The listing builds one solid part. Answer for the finished solid, in the listing's coordinates (mm). A direction names the side the tool comes from. Give positions to 0.01 mm unless a question says otherwise; leave off trailing zeros. Loops run counter-clockwise (first coordinate to the right, second up) from the corner with the lowest first, then second, coordinate; pieces in that order, holes last.
Item 1: A tool of negligible diameter and unlimited length cuts with its end or side. For faces 4 (the face through (2, 34, -2)), 5 (the face through (185.6, 108, -2)), 6 (the face through (205.6, 87, -2)), from which of +Z, -Z, +X, -X, +Y, -Y can it reach the whole face along a straight path? Write none if from no direction.
Item 2: Section B-B, the plane y = 60.12 is taken. Give the vertices of the cut face in (x, z), and give its area (3 significant figures).
Item 3: Section D-D, the plane y = 85 is taken. Give the vertices of the cut face in (x, z).
Item 4: Section C-C, the plane x = 152.65 is taken. Give the vertices of the cut face in (y, z).
Item 5: Section A-A, the plane x = 114 is taken. Give the vertices of the cut face in (y, z), and give its area (3 significant figures).
Item 6: Consider line 1 along X through (y, z) = (55, -2.8); line 2 along X through (y, z) = (101, -1.85); line 3 along X through (y, z) = (92, -0.65). Determine where each line is inside the solid, lowest interval first.
Item 7: The mould has two halves that part along X. Classify faces 1 (the face through (161.6, 108, -2)), 2 (the face through (197, 110, -2)), 3 (the face through (205.6, 23, -2)): pulls with the +X half, pulls with the -X half, needs draft (parallel to the pull), parting line crosses it, or undercut.
Item 8: Each of these flat-tipped pins is pushed along its axis until it touches: pin 1 Ø1.8 at (x, z) = (31, -1.5) entering from -Y; pin 2 Ø1.8 at (x, z) = (1, -1.5) entering from -Y; pin 3 Ø12 at (x, y) = (29.5, 20) entering from +Z; pin 4 Ø1.8 at (x, z) = (171.5, -2) entering from +Y. Where does it stop, or does it pass through?
from build123d import *

# Parameters (mm, degrees)
SKETCH_1_W             = 209.2
SKETCH_1_H             = 110
SM_BASE_FLANGE_1_DEPTH = 3.6
CUT_EXTRUDE_1_REACH    = 238.384
SKETCH_6_W             = 42
SKETCH_6_H             = 21
CUT_EXTRUDE_2_REACH    = 238.384
SKETCH_7_W             = 3.6
SKETCH_7_H             = 22
SKETCH_7_W_2           = 24
SKETCH_7_H_2           = 3.6
SKETCH_7_W_3           = 26
SKETCH_8_R             = 1.6
CUT_EXTRUDE_3_DEPTH    = 10
CUT_EXTRUDE_4_REACH    = 238.384
SKETCH_9_R             = 2.1


# Sheet-metal steps are written as plain solids
with BuildPart() as part:
    # Sketch 1 → Базовая кромка1 (new body)
    with BuildSketch(Plane.XY):
        with Locations((104.6, 55)):
            Rectangle(SKETCH_1_W, SKETCH_1_H)
        with BuildLine():
            Line((17, 12), (139.2, 12))
            ThreePointArc((139.2, 12), (142.735533906, 13.464466094), (144.2, 17))
            Line((144.2, 17), (144.2, 93))
            ThreePointArc((144.2, 93), (142.735533906, 96.535533906), (139.2, 98))
            Line((139.2, 98), (17, 98))
            ThreePointArc((17, 98), (13.464466094, 96.535533906), (12, 93))
            Line((12, 93), (12, 17))
            ThreePointArc((12, 17), (13.464466094, 13.464466094), (17, 12))
        make_face(mode=Mode.SUBTRACT)
    extrude(amount=-SM_BASE_FLANGE_1_DEPTH)

    # Эскиз6 → Вырез-Вытянуть1 (cut, up to next)
    with BuildSketch(Plane.XY, mode=Mode.PRIVATE) as cut_extrude_1_sk1:
        with Locations((176.7, 55)):
            Rectangle(SKETCH_6_W, SKETCH_6_H)
    cut_extrude_1_tool1 = extrude(cut_extrude_1_sk1.sketch, amount=-CUT_EXTRUDE_1_REACH, mode=Mode.PRIVATE) & part.part
    add(cut_extrude_1_tool1.solids().sort_by_distance((176.7, 55, 0))[0], mode=Mode.SUBTRACT)

    # Эскиз7 → Вырез-Вытянуть2 (cut, up to next)
    with BuildSketch(Plane(origin=(0, 0, -3.6), x_dir=(-1, 0, 0), z_dir=(0, 0, -1)), mode=Mode.PRIVATE) as cut_extrude_2_sk1:
        with Locations((-1.8, 87)):
            Rectangle(SKETCH_7_W, SKETCH_7_H)
    cut_extrude_2_tool1 = extrude(cut_extrude_2_sk1.sketch, amount=-CUT_EXTRUDE_2_REACH, mode=Mode.PRIVATE) & part.part
    # Эскиз7 → Вырез-Вытянуть2 (cut, up to next)
    with BuildSketch(Plane(origin=(0, 0, -3.6), x_dir=(-1, 0, 0), z_dir=(0, 0, -1)), mode=Mode.PRIVATE) as cut_extrude_2_sk2:
        with Locations((-35.6, 108.2)):
            Rectangle(SKETCH_7_W_2, SKETCH_7_H_2)
    cut_extrude_2_tool2 = extrude(cut_extrude_2_sk2.sketch, amount=-CUT_EXTRUDE_2_REACH, mode=Mode.PRIVATE) & part.part
    # Эскиз7 → Вырез-Вытянуть2 (cut, up to next)
    with BuildSketch(Plane(origin=(0, 0, -3.6), x_dir=(-1, 0, 0), z_dir=(0, 0, -1)), mode=Mode.PRIVATE) as cut_extrude_2_sk3:
        with Locations((-104.6, 108.2)):
            Rectangle(SKETCH_7_W_3, SKETCH_7_H_2)
    cut_extrude_2_tool3 = extrude(cut_extrude_2_sk3.sketch, amount=-CUT_EXTRUDE_2_REACH, mode=Mode.PRIVATE) & part.part
    # Эскиз7 → Вырез-Вытянуть2 (cut, up to next)
    with BuildSketch(Plane(origin=(0, 0, -3.6), x_dir=(-1, 0, 0), z_dir=(0, 0, -1)), mode=Mode.PRIVATE) as cut_extrude_2_sk4:
        with Locations((-173.6, 108.2)):
            Rectangle(SKETCH_7_W_2, SKETCH_7_H_2)
    cut_extrude_2_tool4 = extrude(cut_extrude_2_sk4.sketch, amount=-CUT_EXTRUDE_2_REACH, mode=Mode.PRIVATE) & part.part
    # Эскиз7 → Вырез-Вытянуть2 (cut, up to next)
    with BuildSketch(Plane(origin=(0, 0, -3.6), x_dir=(-1, 0, 0), z_dir=(0, 0, -1)), mode=Mode.PRIVATE) as cut_extrude_2_sk5:
        with Locations((-207.4, 87)):
            Rectangle(SKETCH_7_W, SKETCH_7_H)
    cut_extrude_2_tool5 = extrude(cut_extrude_2_sk5.sketch, amount=-CUT_EXTRUDE_2_REACH, mode=Mode.PRIVATE) & part.part
    # Эскиз7 → Вырез-Вытянуть2 (cut, up to next)
    with BuildSketch(Plane(origin=(0, 0, -3.6), x_dir=(-1, 0, 0), z_dir=(0, 0, -1)), mode=Mode.PRIVATE) as cut_extrude_2_sk6:
        with Locations((-207.4, 23)):
            Rectangle(SKETCH_7_W, SKETCH_7_H)
    cut_extrude_2_tool6 = extrude(cut_extrude_2_sk6.sketch, amount=-CUT_EXTRUDE_2_REACH, mode=Mode.PRIVATE) & part.part
    # Эскиз7 → Вырез-Вытянуть2 (cut, up to next)
    with BuildSketch(Plane(origin=(0, 0, -3.6), x_dir=(-1, 0, 0), z_dir=(0, 0, -1)), mode=Mode.PRIVATE) as cut_extrude_2_sk7:
        with Locations((-173.6, 1.8)):
            Rectangle(SKETCH_7_W_2, SKETCH_7_H_2)
    cut_extrude_2_tool7 = extrude(cut_extrude_2_sk7.sketch, amount=-CUT_EXTRUDE_2_REACH, mode=Mode.PRIVATE) & part.part
    # Эскиз7 → Вырез-Вытянуть2 (cut, up to next)
    with BuildSketch(Plane(origin=(0, 0, -3.6), x_dir=(-1, 0, 0), z_dir=(0, 0, -1)), mode=Mode.PRIVATE) as cut_extrude_2_sk8:
        with Locations((-104.6, 1.8)):
            Rectangle(SKETCH_7_W_3, SKETCH_7_H_2)
    cut_extrude_2_tool8 = extrude(cut_extrude_2_sk8.sketch, amount=-CUT_EXTRUDE_2_REACH, mode=Mode.PRIVATE) & part.part
    # Эскиз7 → Вырез-Вытянуть2 (cut, up to next)
    with BuildSketch(Plane(origin=(0, 0, -3.6), x_dir=(-1, 0, 0), z_dir=(0, 0, -1)), mode=Mode.PRIVATE) as cut_extrude_2_sk9:
        with Locations((-35.6, 1.8)):
            Rectangle(SKETCH_7_W_2, SKETCH_7_H_2)
    cut_extrude_2_tool9 = extrude(cut_extrude_2_sk9.sketch, amount=-CUT_EXTRUDE_2_REACH, mode=Mode.PRIVATE) & part.part
    # Эскиз7 → Вырез-Вытянуть2 (cut, up to next)
    with BuildSketch(Plane(origin=(0, 0, -3.6), x_dir=(-1, 0, 0), z_dir=(0, 0, -1)), mode=Mode.PRIVATE) as cut_extrude_2_sk10:
        with Locations((-1.8, 23)):
            Rectangle(SKETCH_7_W, SKETCH_7_H)
    cut_extrude_2_tool10 = extrude(cut_extrude_2_sk10.sketch, amount=-CUT_EXTRUDE_2_REACH, mode=Mode.PRIVATE) & part.part
    add(cut_extrude_2_tool1.solids().sort_by_distance((1.8, 87, -3.6))[0], mode=Mode.SUBTRACT)
    add(cut_extrude_2_tool2.solids().sort_by_distance((35.6, 108.2, -3.6))[0], mode=Mode.SUBTRACT)
    add(cut_extrude_2_tool3.solids().sort_by_distance((104.6, 108.2, -3.6))[0], mode=Mode.SUBTRACT)
    add(cut_extrude_2_tool4.solids().sort_by_distance((173.6, 108.2, -3.6))[0], mode=Mode.SUBTRACT)
    add(cut_extrude_2_tool5.solids().sort_by_distance((207.4, 87, -3.6))[0], mode=Mode.SUBTRACT)
    add(cut_extrude_2_tool6.solids().sort_by_distance((207.4, 23, -3.6))[0], mode=Mode.SUBTRACT)
    add(cut_extrude_2_tool7.solids().sort_by_distance((173.6, 1.8, -3.6))[0], mode=Mode.SUBTRACT)
    add(cut_extrude_2_tool8.solids().sort_by_distance((104.6, 1.8, -3.6))[0], mode=Mode.SUBTRACT)
    add(cut_extrude_2_tool9.solids().sort_by_distance((35.6, 1.8, -3.6))[0], mode=Mode.SUBTRACT)
    add(cut_extrude_2_tool10.solids().sort_by_distance((1.8, 23, -3.6))[0], mode=Mode.SUBTRACT)

    # Эскиз8 → Вырез-Вытянуть3 (cut)
    with BuildSketch(Plane(origin=(0, 0, -3.6), x_dir=(-1, 0, 0), z_dir=(0, 0, -1))):
        with Locations((-200.2, 9)):
            Circle(SKETCH_8_R)
        with Locations((-9, 9)):
            Circle(SKETCH_8_R)
        with Locations((-9, 101)):
            Circle(SKETCH_8_R)
        with Locations((-200.2, 101)):
            Circle(SKETCH_8_R)
    extrude(amount=-CUT_EXTRUDE_3_DEPTH, mode=Mode.SUBTRACT)

    # Эскиз9 → Вырез-Вытянуть4 (cut, up to next)
    with BuildSketch(Plane(origin=(0, 0, -3.6), x_dir=(-1, 0, 0), z_dir=(0, 0, -1)), mode=Mode.PRIVATE) as cut_extrude_4_sk1:
        with Locations((-200.91, 60.12)):
            Circle(SKETCH_9_R)
    cut_extrude_4_tool1 = extrude(cut_extrude_4_sk1.sketch, amount=-CUT_EXTRUDE_4_REACH, mode=Mode.PRIVATE) & part.part
    # Эскиз9 → Вырез-Вытянуть4 (cut, up to next)
    with BuildSketch(Plane(origin=(0, 0, -3.6), x_dir=(-1, 0, 0), z_dir=(0, 0, -1)), mode=Mode.PRIVATE) as cut_extrude_4_sk2:
        with Locations((-200.91, 49.96)):
            Circle(SKETCH_9_R)
    cut_extrude_4_tool2 = extrude(cut_extrude_4_sk2.sketch, amount=-CUT_EXTRUDE_4_REACH, mode=Mode.PRIVATE) & part.part
    # Эскиз9 → Вырез-Вытянуть4 (cut, up to next)
    with BuildSketch(Plane(origin=(0, 0, -3.6), x_dir=(-1, 0, 0), z_dir=(0, 0, -1)), mode=Mode.PRIVATE) as cut_extrude_4_sk3:
        with Locations((-152.65, 60.12)):
            Circle(SKETCH_9_R)
    cut_extrude_4_tool3 = extrude(cut_extrude_4_sk3.sketch, amount=-CUT_EXTRUDE_4_REACH, mode=Mode.PRIVATE) & part.part
    # Эскиз9 → Вырез-Вытянуть4 (cut, up to next)
    with BuildSketch(Plane(origin=(0, 0, -3.6), x_dir=(-1, 0, 0), z_dir=(0, 0, -1)), mode=Mode.PRIVATE) as cut_extrude_4_sk4:
        with Locations((-152.65, 49.96)):
            Circle(SKETCH_9_R)
    cut_extrude_4_tool4 = extrude(cut_extrude_4_sk4.sketch, amount=-CUT_EXTRUDE_4_REACH, mode=Mode.PRIVATE) & part.part
    add(cut_extrude_4_tool1.solids().sort_by_distance((200.91, 60.12, -3.6))[0], mode=Mode.SUBTRACT)
    add(cut_extrude_4_tool2.solids().sort_by_distance((200.91, 49.96, -3.6))[0], mode=Mode.SUBTRACT)
    add(cut_extrude_4_tool3.solids().sort_by_distance((152.65, 60.12, -3.6))[0], mode=Mode.SUBTRACT)
    add(cut_extrude_4_tool4.solids().sort_by_distance((152.65, 49.96, -3.6))[0], mode=Mode.SUBTRACT)


solid = part.part
Worked answers:
1. face 4: +Z, -Z, -X
1. face 5: +Z, -Z, +Y
1. face 6: +Z, -Z, +X
2. outline: (0, -3.6) - (12, -3.6) - (12, 0) - (0, 0) - close; (144.2, -3.6) - (150.55, -3.6) - (150.55, 0) - (144.2, 0) - close; (154.75, -3.6) - (155.7, -3.6) - (155.7, 0) - (154.75, 0) - close; (197.7, -3.6) - (198.81, -3.6) - (198.81, 0) - (197.7, 0) - close; (203.01, -3.6) - (209.2, -3.6) - (209.2, 0) - (203.01, 0) - close
2. area: 95.8 mm2
3. outline: (3.6, -3.6) - (12, -3.6) - (12, 0) - (3.6, 0) - close; (144.2, -3.6) - (205.6, -3.6) - (205.6, 0) - (144.2, 0) - close
4. outline: (0, -3.6) - (47.86, -3.6) - (47.86, 0) - (0, 0) - close; (52.06, -3.6) - (58.02, -3.6) - (58.02, 0) - (52.06, 0) - close; (62.22, -3.6) - (110, -3.6) - (110, 0) - (62.22, 0) - close
5. outline: (3.6, -3.6) - (12, -3.6) - (12, 0) - (3.6, 0) - close; (98, -3.6) - (106.4, -3.6) - (106.4, 0) - (98, 0) - close
5. area: 60.5 mm2
6. line 1: x = 0 to 12, 144.2 to 155.7, 197.7 to 209.2
6. line 2: x = 0 to 7.4, 10.6 to 198.6, 201.8 to 209.2
6. line 3: x = 3.6 to 12, 144.2 to 205.6
7. face 1: undercut
7. face 2: needs draft
7. face 3: pulls with the +X half
8. pin 1: stops at y = 3.6
8. pin 2: stops at y = 0
8. pin 3: passes through
8. pin 4: stops at y = 106.4
